Verification items for the finished model (mm, model axes). Give positions to 0.01 mm unless a question says otherwise; leave off trailing zeros. Order: outer loops, then holes, each group sorted by start corner. A loop starts at its lowest first (then second) coordinate and runs counter-clockwise, first axis right, second up.
(1) Gauge pin test, flat ends, axial feed: pin 1 (9 mm diameter, centred on x = 234.95, y = -158.75, fed in from -Z); pin 2 (7.5 mm diameter, centred on x = 24, z = 15.5, fed in from +Y); pin 3 (8 mm diameter, centred on x = 222.25, y = 311.15, fed in from -Z). Record the tip position at first contact, or that the pin passes through.
(2) Scan lines: L1, parallel to Y at x = 190.5, z = 8.25 (3 decimals); L2, parallel to X at y = -24.5, z = 9.75; L3, parallel to X at y = -104, z = 17.5. Record each from-to range of solid material in increasing order.
(3) Sectioned sample at A-A on y = 140.5. Record the cut outline in (x, z) (3 decimals), plus the area to 3 significant figures.
```python
from build123d import *

# Parameters (mm, degrees)
PAD_DEPTH        = 19.05
SKETCH002_W      = 19.05
SKETCH002_H      = 469.9
POCKET001_DEPTH  = 9.525
HOLE_D           = 7.1
HOLE_CSINK_D     = 12.07
HOLE_CSINK_ANGLE = 82
SKETCH005_W      = 25.4
SKETCH005_H      = 431.8
POCKET_DEPTH     = 6.35


with BuildPart() as part:
    # Sketch → Pad (new body)
    with BuildSketch(Plane.XY):
        Polygon((-127, -330.2), (-127, 330.2), (127, 330.2), (127, -139.7), (139.7, -139.7), (139.7, -330.2), align=None)
    pad = extrude(amount=PAD_DEPTH)

    # Sketch002 → Pocket001 (cut)
    with BuildSketch(Plane.XY.offset(19.05)):
        with Locations((22.225, 95.25)):
            Rectangle(SKETCH002_W, SKETCH002_H)
    pocket001 = extrude(amount=-POCKET001_DEPTH, mode=Mode.SUBTRACT)

    # Hole (through all)
    with Locations(Plane(origin=(0, 0, 0), x_dir=(1, 0, 0), z_dir=(0, 0, -1))):
        with Locations((-88.9, 158.75), (88.9, 158.75), (-44.45, 158.75), (44.45, 158.75), (57.15, -311.15), (88.9, -301.625), (114.3, -320.675)):
            hole = CounterSinkHole(HOLE_D / 2, HOLE_CSINK_D / 2, counter_sink_angle=HOLE_CSINK_ANGLE)

    # Sketch005 (on Face5 of Hole) → Pocket (cut)
    with BuildSketch(Plane.XY.offset(19.05)):
        with Locations((114.3, 76.2)):
            Rectangle(SKETCH005_W, SKETCH005_H)
    pocket = extrude(amount=-POCKET_DEPTH, mode=Mode.SUBTRACT)

    # Mirrored: Pad, Pocket001, Hole, Pocket across face of Pocket
    add(pad.mirror(Plane(origin=(139.7, -234.95, 9.525), x_dir=(0, 1, 0), z_dir=(1, 0, 0))))
    add(pocket001.mirror(Plane(origin=(139.7, -234.95, 9.525), x_dir=(0, 1, 0), z_dir=(1, 0, 0))), mode=Mode.SUBTRACT)
    add(hole.mirror(Plane(origin=(139.7, -234.95, 9.525), x_dir=(0, 1, 0), z_dir=(1, 0, 0))), mode=Mode.SUBTRACT)
    add(pocket.mirror(Plane(origin=(139.7, -234.95, 9.525), x_dir=(0, 1, 0), z_dir=(1, 0, 0))), mode=Mode.SUBTRACT)


solid = part.part
```
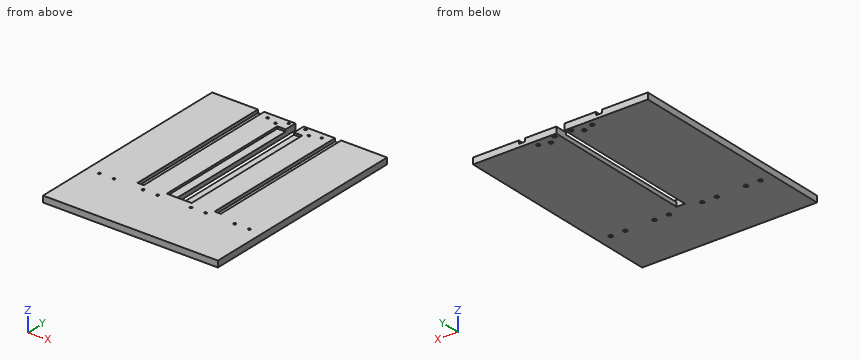
Ans:
1. pin 1: stops at z = 1.77
1. pin 2: stops at y = -139.7
1. pin 3: stops at z = 2.34
2. L1: y = -330.2 to -162.3, -155.2 to 298.075, 305.175 to 330.2
2. L2: x = -127 to 12.7, 31.75 to 127, 152.4 to 247.65, 266.7 to 406.4
2. L3: x = -127 to 12.7, 31.75 to 101.6, 177.8 to 247.65, 266.7 to 406.4
3. outline: (-127, 0) - (127, 0) - (127, 12.7) - (101.6, 12.7) - (101.6, 19.05) - (31.75, 19.05) - (31.75, 9.525) - (12.7, 9.525) - (12.7, 19.05) - (-127, 19.05) - close; (152.4, 0) - (406.4, 0) - (406.4, 19.05) - (266.7, 19.05) - (266.7, 9.525) - (247.65, 9.525) - (247.65, 19.05) - (177.8, 19.05) - (177.8, 12.7) - (152.4, 12.7) - close
3. area: 8,990 mm2
